The listing builds one solid part. Answer for the finished solid, in the listing's coordinates (mm). A direction names the side the tool comes from. Coordinates: 2 decimals unless noted, no trailing zeros. Order: outer loops, then holes, each group sorted by start corner. A loop starts at its lowest first (then second) coordinate and runs counter-clockwise, first axis right, second up. Notation, with made-up numbers: M 21,82 L 57,82 A36 ccw 57,118 Z; hole C 9,76.5 d11. An arc over 180 degrees is marked long. One line per item, written item: value. Start each with the question number.
Q1. For faces 4 (the flat face through (0.6, 0.38, 0)), 5 (the flat face through (7.6, 0.5, -30.5)), determine the directions among +Z, -Z, +X, -X, +Y, -Y from which every point of the face is accessible in a straight line to the end or side of a thin tool.
Q2. The part is cut by section C-C on x = 7.75. Give the vertices of the cut face in (y, z), then the cut area to 3 significant figures.
Q3. Each of these flat-tipped pins is pushed along its axis until it touches: pin 1 Ø8 at (x, z) = (3.5, -21.5) entering from -Y; pin 2 Ø7.5 at (x, z) = (9.5, -23.5) entering from +Y. Where does it stop, or does it pass through?
Q4. Straight lines are drawn through the part: line 1 along X through (y, z) = (0.3, -8.5); line 2 along X through (y, z) = (0.9, -16); line 3 along Z through (x, y) = (7.75, 0.95). For each, find the intervals that lie inside material, in ascending order. Write a range as [from, to].
Q5. The part is cut by section A-A on z = -23.5. Give the vertices of the cut face in (x, y).
Q6. The part is cut by section B-B on y = 0.2. Give the vertices of the cut face in (x, z).
Q7. Determine the mould class of faces 1 (the flat face through (1, 0.5, -15.5)), 2 (the flat face through (14.38, 0.38, 0)), 3 (the flat face through (14, 0.5, -15)) for opening direction X: pulls with the +X half, pulls with the -X half, needs draft (parallel to the pull), parting line crosses it, or undercut.
Autodesk Fusion 360 part; units mm, degrees
sketch "Sketch1" plane through (0, 0, 0) normal (0, 1, 0) x (1, 0, 0)
  line L0 (0, 0) -> (15, 0)
  line L1 (15, 0) -> (15, 31.5)
  line L2 (15, 31.5) -> (0, 31.5)
  line L3 (0, 31.5) -> (0, 0)
  line L4 (1, 0) -> (14, 0)
  line L5 (14, 0) -> (14, 30.5)
  line L6 (14, 30.5) -> (1, 30.5)
  line L7 (1, 30.5) -> (1, 0)
  line L8 (0.5, 0) -> (14.5, 0)
  line L9 (14.5, 0) -> (14.5, 31)
  line L10 (14.5, 31) -> (0.5, 31)
  line L11 (0.5, 31) -> (0.5, 0)
  dimension "d1" = 15
  dimension "d2" = 31.5
  dimension "d3" = 13
  dimension "d4" = 30.5
  dimension "d5" = 1
  dimension "d6" = 14
  dimension "d7" = 31
  dimension "d8" = 0.5
extrude "Extrude1" add sketch "Sketch1" along normal blind 0.5 contours L0 L1 L2 L3 L9 L10 L11
extrude "Extrude2" add sketch "Sketch1" along normal blind 1 contours L0 L5 L6 L7 L8 L9 L10 L11
Output:
1. face 4: +Z, +X, -X, +Y, -Y
1. face 5: +Z, +Y, -Y
2. outline: M 0,-31.5 L 0.5,-31.5 L 0.5,-31 L 1,-31 L 1,-30.5 L 0,-30.5 Z
2. area: 0.750 mm^2
3. pin 1: stops at y = 0
3. pin 2: passes through
4. line 1: x = [0, 1], [14, 15]
4. line 2: x = [0.5, 1], [14, 14.5]
4. line 3: z = [-31, -30.5]
5. outline: M 0,0 L 1,0 L 1,1 L 0.5,1 L 0.5,0.5 L 0,0.5 Z; M 14,0 L 15,0 L 15,0.5 L 14.5,0.5 L 14.5,1 L 14,1 Z
6. outline: M 0,-31.5 L 15,-31.5 L 15,0 L 14,0 L 14,-30.5 L 1,-30.5 L 1,0 L 0,0 Z
7. face 1: undercut
7. face 2: needs draft
7. face 3: undercut
